```python
from build123d import *

# Parameters (mm, degrees)
SKETCH1_W           = 2.9
SKETCH1_H           = 20
BOSS_EXTRUDE1_DEPTH = 5
CUT_EXTRUDE1_DEPTH  = 6
FILLET1_R           = 10
SKETCH3_W           = 3
SKETCH3_H           = 19.8
CUT_EXTRUDE2_DEPTH  = 5
LPATTERN1_COUNT     = 2
LPATTERN1_PITCH     = 80
CUT_EXTRUDE3_DEPTH  = 10
CUT_EXTRUDE4_DEPTH  = 5
BOSS_EXTRUDE2_DEPTH = 5
BOSS_EXTRUDE3_DEPTH = 5
FILLET3_R           = 10
FILLET4_R           = 5
SKETCH12_W          = 20
SKETCH12_H          = 5
BOSS_EXTRUDE4_DEPTH = 5
SKETCH13_R          = 7.5
CUT_EXTRUDE6_DEPTH  = 6


with BuildPart() as part:
    # Sketch1 → Boss-Extrude1 (new body)
    with BuildSketch(Plane.XY):
        with BuildLine():
            Line((155, 62.071067812), (155, 65.538881442))
            ThreePointArc((155, 65.538881442), (153.730862151, 68.867645118), (150.567732956, 70.506544805))
            Line((150.567732956, 70.506544805), (34.432267044, 83.779169481))
            ThreePointArc((34.432267044, 83.779169481), (31.269137849, 85.418069168), (30, 88.746832844))
            Line((30, 88.746832844), (30, 260))
            Line((30, 260), (25, 260))
            Line((25, 260), (25, 263))
            Line((25, 263), (5, 263))
            Line((5, 263), (5, 260))
            Line((5, 260), (0, 260))
            Line((0, 260), (0, 0))
            Line((0, 0), (5, 0))
            Line((5, 0), (5, -5))
            Line((5, -5), (25, -5))
            Line((25, -5), (25, 0))
            Line((25, 0), (30, 0))
            Line((30, 0), (30, 40))
            ThreePointArc((30, 40), (31.464466094, 43.535533906), (35, 45))
            Line((35, 45), (105, 45))
            ThreePointArc((105, 45), (108.535533906, 43.535533906), (110, 40))
            Line((110, 40), (110, 0))
            Line((110, 0), (115, 0))
            Line((115, 0), (115, -5))
            Line((115, -5), (135, -5))
            Line((135, -5), (135, 0))
            Line((135, 0), (140, 0))
            Line((140, 0), (140, 42.928932188))
            ThreePointArc((140, 42.928932188), (140.380602337, 44.84234935), (141.464466094, 46.464466094))
            Line((141.464466094, 46.464466094), (153.535533906, 58.535533906))
            ThreePointArc((153.535533906, 58.535533906), (154.619397663, 60.15765065), (155, 62.071067812))
        make_face()
        with Locations((38.6, 62)):
            Rectangle(SKETCH1_W, SKETCH1_H, mode=Mode.SUBTRACT)
        with Locations((48.6, 62)):
            Rectangle(SKETCH1_W, SKETCH1_H, mode=Mode.SUBTRACT)
        with Locations((118.6, 62)):
            Rectangle(SKETCH1_W, SKETCH1_H, mode=Mode.SUBTRACT)
        with Locations((108.6, 62)):
            Rectangle(SKETCH1_W, SKETCH1_H, mode=Mode.SUBTRACT)
    extrude(amount=BOSS_EXTRUDE1_DEPTH)

    # Sketch2 → Cut-Extrude1 (cut, through all)
    with BuildSketch(Plane.XY.offset(5)):
        with BuildLine():
            Line((30, 40), (30, 48))
            Line((30, 48), (110, 48))
            Line((110, 48), (110, 40))
            ThreePointArc((110, 40), (108.535533906, 43.535533906), (105, 45))
            Line((105, 45), (35, 45))
            ThreePointArc((35, 45), (31.464466094, 43.535533906), (30, 40))
        make_face()
    extrude(amount=-CUT_EXTRUDE1_DEPTH, mode=Mode.SUBTRACT)

    # Fillet1
    fillet1_edges = [part.edges().sort_by_distance(p)[0] for p in [
        (30, 48, 2.5),
        (110, 48, 2.5),
    ]]
    fillet(fillet1_edges, radius=FILLET1_R)

    # Sketch3 → Cut-Extrude2 (cut)
    with BuildSketch(Plane(origin=(0, 0, 0), x_dir=(-1, 0, 0), z_dir=(0, 0, -1))):
        with Locations((-1.5, 200.1)):
            Rectangle(SKETCH3_W, SKETCH3_H)
    cut_extrude2 = extrude(amount=-CUT_EXTRUDE2_DEPTH, mode=Mode.SUBTRACT)

    # LPattern1: Cut-Extrude2 ×2
    with Locations(*[(0, -i * LPATTERN1_PITCH, 0) for i in range(1, LPATTERN1_COUNT)]):
        add(cut_extrude2, mode=Mode.SUBTRACT)

    # Sketch4 → Cut-Extrude3 (cut)
    with BuildSketch(Plane.XY.offset(5)):
        with BuildLine():
            Line((30, 88.746832844), (30, 75))
            Line((30, 75), (111.25, 75))
            Line((111.25, 75), (34.432267044, 83.779169481))
            ThreePointArc((34.432267044, 83.779169481), (31.269137849, 85.418069168), (30, 88.746832844))
        make_face()
    extrude(amount=-CUT_EXTRUDE3_DEPTH, mode=Mode.SUBTRACT)

    # Sketch5 → Cut-Extrude4 (cut)
    with BuildSketch(Plane.XY.offset(5)):
        with BuildLine():
            Line((150.567732956, 70.506544805), (134.9100099, 72.295998869))
            Line((134.9100099, 72.295998869), (153.535533906, 58.535533906))
            ThreePointArc((153.535533906, 58.535533906), (154.619397663, 60.15765065), (155, 62.071067812))
            Line((155, 62.071067812), (155, 65.538881442))
            ThreePointArc((155, 65.538881442), (153.730862151, 68.867645118), (150.567732956, 70.506544805))
        make_face()
    extrude(amount=-CUT_EXTRUDE4_DEPTH, mode=Mode.SUBTRACT)

    # Sketch5<3> → Boss-Extrude2 (add)
    with BuildSketch(Plane.XY.offset(5)):
        Polygon((131.25, 75), (111.25, 75), (134.9100099, 72.295998869), align=None)
    extrude(amount=-BOSS_EXTRUDE2_DEPTH)

    # Sketch10 → Boss-Extrude3 (add)
    with BuildSketch(Plane(origin=(0, 0, 0), x_dir=(-1, 0, 0), z_dir=(0, 0, -1))):
        Polygon((-131.25, 75), (-200, 42.941348502), (-200, 0), (-170, 0), (-170, 48), (-143, 48), (-153.535533906, 58.535533906), align=None)
    extrude(amount=-BOSS_EXTRUDE3_DEPTH)

    # Fillet3
    fillet3_edges = [part.edges().sort_by_distance(p)[0] for p in [
        (131.25, 75, 2.5),
        (170, 48, 2.5),
    ]]
    fillet(fillet3_edges, radius=FILLET3_R)

    # Fillet4
    fillet4_edges = [part.edges().sort_by_distance(p)[0] for p in [
        (200, 42.941348502, 2.5),
    ]]
    fillet(fillet4_edges, radius=FILLET4_R)

    # Sketch12 → Boss-Extrude4 (add)
    with BuildSketch(Plane.XY.offset(5)):
        with Locations((185, -2.5)):
            Rectangle(SKETCH12_W, SKETCH12_H)
    extrude(amount=-BOSS_EXTRUDE4_DEPTH)

    # Sketch13 → Cut-Extrude6 (cut, through all)
    with BuildSketch(Plane.XY.offset(5)):
        with Locations((15, 20)):
            Circle(SKETCH13_R)
        with Locations((125, 20)):
            Circle(SKETCH13_R)
        with Locations((185, 20)):
            Circle(SKETCH13_R)
    extrude(amount=-CUT_EXTRUDE6_DEPTH, mode=Mode.SUBTRACT)


solid = part.part
```
Read the model definition and answer for the solid it produces. Units are mm, in the model's axes. A direction names the side the tool comes from. Round coordinates to 2 decimals unless told otherwise and drop trailing zeros. Write each loop counter-clockwise with the first axis right and the second up, starting at its lowest first coordinate (ties: lowest second). Pieces come first, ordered by that corner, then holes. Notation, with made-up numbers: (-30, 27.25) -> (-2, 27.25) arc R17 cw to (-2, 55.25) -> close; hole circle Ø7 at (-23.75, -30). An arc over 180 degrees is marked (long way). Answer in a Markdown table with one row per item. Add a question column.
1) Find section C-C, the plane z = 0.9. State how many separate pieces and enclosed holes the cut face has, and give its area (3 significant figures).
2) Consider line 1 (X direction, y = 30.5, z = 3.7); line 2 (Y direction, x = 125, z = 1.45); line 3 (Y direction, x = 53.5, z = 1.35). Determine where each line is inside the solid, lowest interval first.
3) Find section B-B, the plane y = 20. Determine the outline of the cut face in (x, z), and give its area (3 significant figures).
4) Find section D-D, the plane y = 216.5. Determine the outline of the cut face in (x, z).
5) Find section A-A, the plane x = 125. Determine the outline of the cut face in (y, z).
6) Determine the mould class of faces 1 (the face through (63, 70, 5)), 2 (the face through (14.024, 27.436, 2.535)), 3 (the face through (33.01, 45.15, 2.46)) for opening direction Y: pulls with the +Y half, pulls with the -Y half, needs draft (parallel to the pull), parting line crosses it, or undercut.
7) Which of the six approach directions +Z, -Z, +X, -X, +Y, -Y give full straight-line access (tool end or side, diameter ignored) to faces 4 (the face through (167.15, 44.99, 2.54)), 5 (the face through (132.154, 22.253, 2.535))?
8) Given P1, Ø1.5, axis at y = 168.5, z = 3, coming from the +X side; P2, Ø1.5, axis at x = 42.5, z = 1, coming from the -Y side; P3, Ø1.5, axis at y = 60.5, z = 2, coming from the +X side; P4, Ø12, axis at x = 125, y = 20, coming from the -Z side, each flat-ended and moving along its own axis, determine where each tip first touches the part or whether it passes through.
Findings below:
| question | item | result |
|---|---|---|
| 1 | separate pieces | 1 |
| 1 | enclosed holes | 7 |
| 1 | area | 13,700 mm² |
| 2 | line 1 | 0 to 30, 110 to 140, 170 to 200 |
| 2 | line 2 | -5 to 12.5, 27.5 to 75 |
| 2 | line 3 | 48 to 75 |
| 3 | outline | (0, 0) -> (7.5, 0) -> (7.5, 5) -> (0, 5) -> close; (22.5, 0) -> (30, 0) -> (30, 5) -> (22.5, 5) -> close; (110, 0) -> (117.5, 0) -> (117.5, 5) -> (110, 5) -> close; (132.5, 0) -> (140, 0) -> (140, 5) -> (132.5, 5) -> close; (170, 0) -> (177.5, 0) -> (177.5, 5) -> (170, 5) -> close; (192.5, 0) -> (200, 0) -> (200, 5) -> (192.5, 5) -> close |
| 3 | area | 225 mm² |
| 4 | outline | (0, 0) -> (30, 0) -> (30, 5) -> (0, 5) -> close |
| 5 | outline | (-5, 0) -> (12.5, 0) -> (12.5, 5) -> (-5, 5) -> close; (27.5, 0) -> (75, 0) -> (75, 5) -> (27.5, 5) -> close |
| 6 | face 1 | needs draft |
| 6 | face 2 | undercut |
| 6 | face 3 | pulls with the -Y half |
| 7 | face 4 | +Z, -Z, -Y |
| 7 | face 5 | +Z, -Z |
| 8 | P1 | x = 30 |
| 8 | P2 | y = 48 |
| 8 | P3 | x = 163.95 |
| 8 | P4 | through |
